The model under review builds one solid part; all positions refer to its coordinate system, in mm. A direction names the side the tool comes from. Round coordinates to 2 decimals unless told otherwise and drop trailing zeros. Order: outer loops, then holes, each group sorted by start corner. A loop starts at its lowest first (then second) coordinate and runs counter-clockwise, first axis right, second up. Notation, with made-up numbers: (14, 8) - (60, 8) arc R14 cw to (60, 15) - close; hole circle Ø10 at (50, -2.5). An arc over 180 degrees is marked (long way). One line per question, with ' | ' between items. Start each with the question number.
Item 1: Add section B-B on y = -10. State the section outline as (x, z) points.
Item 2: Add section C-C on x = -3.5. State the section outline as (y, z) points, and give its area (3 significant figures).
Item 3: Add section D-D on z = 26. State the section outline as (x, y) points.
Item 4: Tool access review of faces 1 (the face through (-33, -41, 10)), 2 (the face through (-25, 0, 2)), 3 (the face through (-66, -80, 60)), 4 (the face through (-25, 0, 97)), 5 (the face through (-68, -35, 75)): name each direction out of +Z, -Z, +X, -X, +Y, -Y from which nothing blocks a thin tool from reaching the whole face with its end or side.
Item 5: Draft analysis for pull direction Z (two halves, no side actions). For faces 6 (the face through (-35, 5, 51)), 7 (the face through (-25, 3, 100)), 8 (the face through (-48.699, 2.535, 29.143)), state which applies: +Z half, -Z half, draft (parallel to the pull), parting line (faces both ways), or undercut.
Item 6: Insertion check: pin 1 Ø12 at (x, y) = (-51.5, -33.5) entering from +Z; pin 2 Ø19.5 at (x, z) = (-39, 51) entering from -Y; pin 3 Ø5.5 at (y, z) = (2, 98.5) entering from -X; pin 4 Ø15.5 at (x, z) = (-50, 35) entering from +Y. Each pin has a flat end and moves straight along its axis. Give the tip position at first contact, or say it passes through.
Item 7: For L1, parallel to Y at x = -66, z = 50 (3 decimals); L2, parallel to Z at x = -53, y = -66.5; L3, parallel to Y at x = -45.5, z = 78, list the stretches that pass through material, from the lowest coordinate up. Write a range as [from, to].
Item 8: Add section A-A on z = 43. State the section outline as (x, y) points (3 decimals).
from build123d import *

# Parameters (mm, degrees)
BOSS_EXTRUDE1_DEPTH = 100
SKETCH2_W           = 5
SKETCH2_H           = 80
CUT_EXTRUDE2_DEPTH  = 5
SKETCH3_W           = 5
SKETCH3_H           = 80
CUT_EXTRUDE3_DEPTH  = 5
SKETCH4_W           = 15
SKETCH4_H           = 5
CUT_EXTRUDE4_DEPTH  = 5
SKETCH5_W           = 15
SKETCH5_H           = 5
CUT_EXTRUDE5_DEPTH  = 5
SKETCH6_R           = 1.5
CUT_EXTRUDE6_DEPTH  = 10
SKETCH7_W           = 66.05
SKETCH7_H           = 42.1
CUT_EXTRUDE7_DEPTH  = 10
SKETCH8_W           = 5
SKETCH8_H           = 20
BOSS_EXTRUDE2_DEPTH = 42.1
SKETCH10_R          = 6
CUT_EXTRUDE8_DEPTH  = 5
SKETCH11_W          = 5
SKETCH11_H          = 25
CUT_EXTRUDE9_DEPTH  = 100
SKETCH12_W          = 5
SKETCH12_H          = 5
CUT_EXTRUDE10_DEPTH = 5
SKETCH13_W          = 5
SKETCH13_H          = 5
CUT_EXTRUDE11_DEPTH = 5
SKETCH14_W          = 5
SKETCH14_H          = 80
BOSS_EXTRUDE3_DEPTH = 65


with BuildPart() as part:
    # Sketch1 → Boss-Extrude1 (new body)
    with BuildSketch(Plane.XY):
        Polygon((0, 0), (-65, 0), (-65, -80), (-70, -80), (-70, 0), (-70, 30), (-65, 30), (-65, 5), (0, 5), align=None)
    extrude(amount=BOSS_EXTRUDE1_DEPTH)

    # Sketch2 → Cut-Extrude2 (cut)
    with BuildSketch(Plane.XY.offset(100)):
        with Locations((-67.5, -40)):
            Rectangle(SKETCH2_W, SKETCH2_H)
    extrude(amount=-CUT_EXTRUDE2_DEPTH, mode=Mode.SUBTRACT)

    # Sketch3 → Cut-Extrude3 (cut)
    with BuildSketch(Plane(origin=(0, 0, 0), x_dir=(-1, 0, 0), z_dir=(0, 0, -1))):
        with Locations((67.5, -40)):
            Rectangle(SKETCH3_W, SKETCH3_H)
    extrude(amount=-CUT_EXTRUDE3_DEPTH, mode=Mode.SUBTRACT)

    # Sketch4 → Cut-Extrude4 (cut)
    with BuildSketch(Plane.XY.offset(100)):
        with Locations((-57.5, 2.5)):
            Rectangle(SKETCH4_W, SKETCH4_H)
    extrude(amount=-CUT_EXTRUDE4_DEPTH, mode=Mode.SUBTRACT)

    # Sketch5 → Cut-Extrude5 (cut)
    with BuildSketch(Plane(origin=(0, 0, 0), x_dir=(-1, 0, 0), z_dir=(0, 0, -1))):
        with Locations((57.5, 2.5)):
            Rectangle(SKETCH5_W, SKETCH5_H)
    extrude(amount=-CUT_EXTRUDE5_DEPTH, mode=Mode.SUBTRACT)

    # Sketch6 → Cut-Extrude6 (cut)
    with BuildSketch(Plane(origin=(-65, 0, 0), x_dir=(0, 0, -1), z_dir=(1, 0, 0))):
        with Locations((-50, -10)):
            Circle(SKETCH6_R)
        with Locations((-50, -60.45)):
            Circle(SKETCH6_R)
    extrude(amount=-CUT_EXTRUDE6_DEPTH, mode=Mode.SUBTRACT)

    # Sketch7 → Cut-Extrude7 (cut)
    with BuildSketch(Plane(origin=(-65, 0, 0), x_dir=(0, 0, -1), z_dir=(1, 0, 0))):
        with Locations((-61.975, -35.225)):
            Rectangle(SKETCH7_W, SKETCH7_H)
    extrude(amount=-CUT_EXTRUDE7_DEPTH, mode=Mode.SUBTRACT)

    # Sketch8 → Boss-Extrude2 (add)
    with BuildSketch(Plane.XZ.offset(14.175)):
        with Locations((-67.5, 85)):
            Rectangle(SKETCH8_W, SKETCH8_H)
    extrude(amount=BOSS_EXTRUDE2_DEPTH)

    # Sketch10 → Cut-Extrude8 (cut)
    with BuildSketch(Plane(origin=(0, 5, 0), x_dir=(1, 0, 0), z_dir=(0, 1, 0))):
        with Locations(Location((-50, -35, 0), (0, 0, 180))):
            Circle(SKETCH10_R)
    extrude(amount=-CUT_EXTRUDE8_DEPTH, mode=Mode.SUBTRACT)

    # Sketch11 → Cut-Extrude9 (cut)
    with BuildSketch(Plane.XY.offset(100)):
        with Locations((-67.5, 17.5)):
            Rectangle(SKETCH11_W, SKETCH11_H)
    extrude(amount=-CUT_EXTRUDE9_DEPTH, mode=Mode.SUBTRACT)

    # Sketch12 → Cut-Extrude10 (cut)
    with BuildSketch(Plane.XY.offset(100)):
        with Locations((-67.5, 2.5)):
            Rectangle(SKETCH12_W, SKETCH12_H)
    extrude(amount=-CUT_EXTRUDE10_DEPTH, mode=Mode.SUBTRACT)

    # Sketch13 → Cut-Extrude11 (cut)
    with BuildSketch(Plane(origin=(0, 0, 0), x_dir=(-1, 0, 0), z_dir=(0, 0, -1))):
        with Locations((67.5, 2.5)):
            Rectangle(SKETCH13_W, SKETCH13_H)
    extrude(amount=-CUT_EXTRUDE11_DEPTH, mode=Mode.SUBTRACT)

    # Sketch14 → Boss-Extrude3 (add)
    with BuildSketch(Plane(origin=(-65, 0, 0), x_dir=(0, 0, -1), z_dir=(1, 0, 0))):
        with Locations((-92.5, -40)):
            Rectangle(SKETCH14_W, SKETCH14_H)
        with Locations((-7.5, -40)):
            Rectangle(SKETCH14_W, SKETCH14_H)
    extrude(amount=BOSS_EXTRUDE3_DEPTH)


solid = part.part
Determined:
1) outline: (-70, 5) - (0, 5) - (0, 10) - (-65, 10) - (-65, 48.5) - (-70, 48.5) - close; (-70, 51.5) - (-65, 51.5) - (-65, 90) - (0, 90) - (0, 95) - (-70, 95) - close
2) outline: (-80, 5) - (0, 5) - (0, 0) - (5, 0) - (5, 100) - (0, 100) - (0, 95) - (-80, 95) - (-80, 90) - (0, 90) - (0, 10) - (-80, 10) - close | area: 1,300 mm2
3) outline: (-70, -80) - (-65, -80) - (-65, 0) - (0, 0) - (0, 5) - (-70, 5) - close
4) face 1: +X, -Y | face 2: -Z, +X, -X, -Y | face 3: +Z, -Z, +X, -X, -Y | face 4: +Z, +X, -X, -Y | face 5: +X, -X
5) face 6: draft | face 7: +Z half | face 8: undercut
6) pin 1: z = 95 | pin 2: y = 0 | pin 3: x = -50 | pin 4: y = 5
7) L1: [-80, -61.95], [-58.95, -56.275], [-14.175, -11.5], [-8.5, 5] | L2: [5, 10], [90, 95] | L3: [0, 5]
8) outline: (-70, -80) - (-65, -80) - (-65, -56.275) - (-70, -56.275) - close; (-70, -14.175) - (-65, -14.175) - (-65, 0) - (0, 0) - (0, 5) - (-70, 5) - close
